Could you check a few things on this model? Use its own coordinates, in mm. Round coordinates to 2 decimals unless told otherwise and drop trailing zeros. Loops run counter-clockwise (first coordinate to the right, second up) from the corner with the lowest first, then second, coordinate; pieces in that order, holes last. Notation, with made-up numbers: (8, -23.5) -> (16, -23.5) arc R21 cw to (16, -10.5) -> close; hole circle Ø11 at (-31.75, 89). An arc over 180 degrees is marked (long way). Write each question's results on one line, items separated by ' | '. Start each with the question number.
1) Imagine slicing it at B-B, the plane z = 28.25. List the corners of the cut face in (x, y) for me, plus the area to 3 significant figures.
2) For P1, Ø1, axis at y = -1, z = 19, coming from the +X side; P2, Ø2, axis at y = -3, z = 26.5, coming from the +X side, each with a flat end and sliding along its axis, tell me the tip position at first contact or that it passes through.
3) Imagine slicing it at C-C, the plane z = 17.75. List the corners of the cut face in (x, y) for me, plus the area to 3 significant figures.
4) Imagine slicing it at A-A, the plane y = -0.8. List the corners of the cut face in (x, z) for me, plus the area to 3 significant figures.
5) If I drill on probe 1 along X at (y, z) = (-1.4, 23); probe 2 along X at (y, z) = (-3.3, 21.25); probe 3 along X at (y, z) = (-0.6, 28.25), over which ranges is the centre line in solid material (lowest first)?
from build123d import *

# Parameters (mm, degrees)
F0_W     = 94.0563417971
F0_H     = 12.6443672925
F0_R     = 2.0927521529
F1_DEPTH = 5
F2_R     = 5


# Not quite as in the source:
# - the program builds the solid bodies; features that only make, move or delete a surface that nothing else refers to are left out


with BuildPart() as f1:
    # F0 (on Front) → F1 (new body)
    with BuildSketch(Plane.XZ):
        with Locations((-9.9823940545, 22.7376772091)):
            Rectangle(F0_W, F0_H)
        with Locations((-51.6735911369, 21.9417177141)):
            Circle(F0_R, mode=Mode.SUBTRACT)
    extrude(amount=F1_DEPTH)

    # F2
    f2_edges = [f1.edges().sort_by_distance(p)[0] for p in [
        (37.045777, -2.5, 29.059861),
        (37.045777, -2.5, 16.415494),
        (-57.010565, -2.5, 16.415494),
        (-57.010565, -2.5, 29.059861),
    ]]
    fillet(f2_edges, radius=F2_R)


solid = f1.part
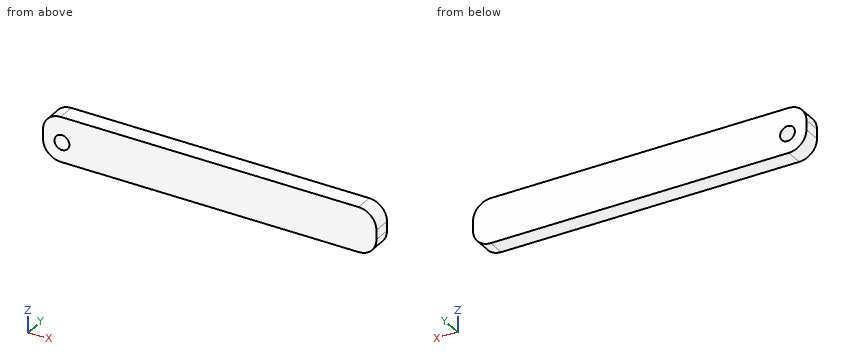
Checked values:
1) outline: (-54.74, -5) -> (34.77, -5) -> (34.77, 0) -> (-54.74, 0) -> close | area: 448 mm^2
2) P1: x = 36.66 | P2: x = 36.83
3) outline: (-55.41, -5) -> (35.45, -5) -> (35.45, 0) -> (-55.41, 0) -> close | area: 454 mm^2
4) outline: (-57.01, 21.42) arc R5 ccw to (-52.01, 16.42) -> (32.05, 16.42) arc R5 ccw to (37.05, 21.42) -> (37.05, 24.06) arc R5 ccw to (32.05, 29.06) -> (-52.01, 29.06) arc R5 ccw to (-57.01, 24.06) -> close; hole circle Ø4.19 at (-51.67, 21.94) | area: 1,150 mm^2
5) probe 1: -57.01 to -53.48, -49.87 to 37.05 | probe 2: -57.01 to -53.65, -49.7 to 37.04 | probe 3: -54.74 to 34.77
